Read the model definition and answer for the solid it produces. Units are mm, in the model's axes. Face numbers are marked on the shaded views. A direction names the side the tool comes from. Coordinates: 2 decimals unless noted, no trailing zeros. Write each loop counter-clockwise with the first axis right and the second up, starting at its lowest first coordinate (ties: lowest second). Pieces come first, ordered by that corner, then holes.
(1) Section A-A on y = 89 is taken. Write down the section's boundary in (x, z).
(2) Section D-D on z = 58.5 is taken. Write down the section's boundary in (x, y).
(3) The mould has two halves that part along Z. Classify the marked faces 1, 2 and 3: +Z half, -Z half, draft (parallel to the pull), parting line (faces both ways), or undercut.
(4) Section C-C on z = 45.5 is taken. Write down the section's boundary in (x, y), then the cut area to 3 significant figures.
(5) Section B-B on x = 27 is taken. Write down the section's boundary in (y, z), then the cut area to 3 significant figures.
(6) Which of the six approach directions +Z, -Z, +X, -X, +Y, -Y give full straight-line access (tool end or side, diameter ignored) to the marked faces 4 and 5?
(7) Find the intervals of material crossed by probe 1 along Z at (x, y) = (72, 8); probe 2 along Z at (x, y) = (38, 95.5); probe 3 along Y at (x, z) = (84, 46.5), in increasing order.
from build123d import *

# Parameters (mm, degrees)
F0_W     = 50.8
F0_H     = 25.4
F1_DEPTH = 203.2


with BuildPart() as f1:
    # F0 (on Right) → F1 (new body)
    with BuildSketch(Plane.YZ):
        Polygon((0, 63.5), (25.4, 38.1), (25.4, 63.5), align=None)
        with Locations((50.8, 50.8)):
            Rectangle(F0_W, F0_H)
        Polygon((76.2, 63.5), (76.2, 38.1), (101.6, 63.5), align=None)
        Polygon((0, 38.1), (0, 0), (101.6, 0), (101.6, 38.1), (76.2, 38.1), (25.4, 38.1), align=None)
    extrude(amount=F1_DEPTH)


solid = f1.part
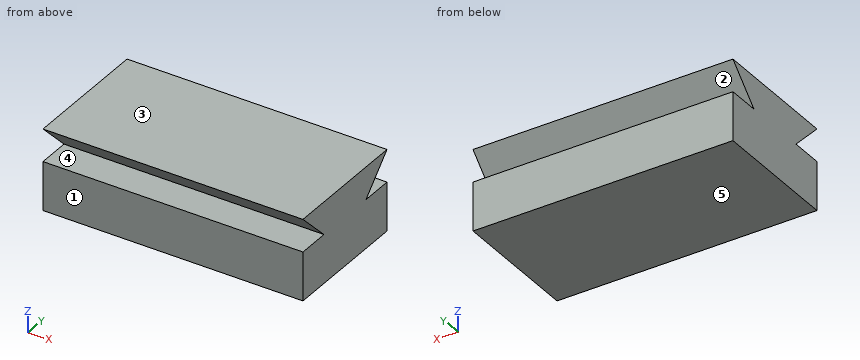
Response:
1. outline: (0, 0) - (203.2, 0) - (203.2, 38.1) - (0, 38.1) - close; (0, 50.9) - (203.2, 50.9) - (203.2, 63.5) - (0, 63.5) - close
2. outline: (0, 5) - (203.2, 5) - (203.2, 96.6) - (0, 96.6) - close
3. face 1: draft
3. face 2: undercut
3. face 3: +Z half
4. outline: (0, 18) - (203.2, 18) - (203.2, 83.6) - (0, 83.6) - close
4. area: 13,300 mm2
5. outline: (0, 0) - (101.6, 0) - (101.6, 38.1) - (76.2, 38.1) - (101.6, 63.5) - (0, 63.5) - (25.4, 38.1) - (0, 38.1) - close
5. area: 5,810 mm2
6. face 4: +X, -X, -Y
6. face 5: -Z, +X, -X, +Y, -Y
7. probe 1: z = 0 to 38.1, 55.5 to 63.5
7. probe 2: z = 0 to 38.1, 57.4 to 63.5
7. probe 3: y = 17 to 84.6
